```python
from build123d import *

# Parameters (mm, degrees)
SKETCH1_W           = 20
SKETCH1_H           = 15
BOSS_EXTRUDE1_DEPTH = 4.5
SKETCH3_R           = 1.6
CUT_EXTRUDE1_DEPTH  = 20
SKETCH4_W           = 1
SKETCH4_H           = 15
CUT_EXTRUDE2_DEPTH  = 2.5
SKETCH5_W           = 1
SKETCH5_H           = 15
CUT_EXTRUDE3_DEPTH  = 2.5
SKETCH6_W           = 1
SKETCH6_H           = 15
CUT_EXTRUDE5_DEPTH  = 2.5


with BuildPart() as part:
    # Sketch1 → Boss-Extrude1 (new body)
    with BuildSketch(Plane(origin=(0, 0, 0), x_dir=(1, 0, 0), z_dir=(0, 1, 0))):
        Rectangle(SKETCH1_W, SKETCH1_H)
    extrude(amount=BOSS_EXTRUDE1_DEPTH)

    # Sketch3 → Cut-Extrude1 (cut)
    with BuildSketch(Plane(origin=(10, 0, 0), x_dir=(0, 0, -1), z_dir=(1, 0, 0))):
        with Locations((0, 3.72608181)):
            Circle(SKETCH3_R)
    extrude(amount=-CUT_EXTRUDE1_DEPTH, mode=Mode.SUBTRACT)

    # Sketch4 → Cut-Extrude2 (cut)
    with BuildSketch(Plane(origin=(0, 4.5, 0), x_dir=(1, 0, 0), z_dir=(0, 1, 0))):
        with Locations((-7.162357261, 0)):
            Rectangle(SKETCH4_W, SKETCH4_H)
    extrude(amount=-CUT_EXTRUDE2_DEPTH, mode=Mode.SUBTRACT)

    # Sketch5 → Cut-Extrude3 (cut)
    with BuildSketch(Plane(origin=(0, 4.5, 0), x_dir=(1, 0, 0), z_dir=(0, 1, 0))):
        with Locations((-4.526212298, 0)):
            Rectangle(SKETCH5_W, SKETCH5_H)
    extrude(amount=-CUT_EXTRUDE3_DEPTH, mode=Mode.SUBTRACT)

    # Sketch6 → Cut-Extrude5 (cut)
    with BuildSketch(Plane(origin=(0, 4.5, 0), x_dir=(1, 0, 0), z_dir=(0, 1, 0))):
        with Locations((-1.483369352, 0)):
            Rectangle(SKETCH6_W, SKETCH6_H)
    extrude(amount=-CUT_EXTRUDE5_DEPTH, mode=Mode.SUBTRACT)


solid = part.part
```
Here's how the part is built. I have some questions about the finished solid (model axes, mm). A direction names the side the tool comes from. Give positions to 0.01 mm unless a question says otherwise; leave off trailing zeros. Loops run counter-clockwise (first coordinate to the right, second up) from the corner with the lowest first, then second, coordinate; pieces in that order, holes last. Notation, with made-up numbers: M 44,24 L 95,24 A23 ccw 95,34 Z; hole C 66,2 d4. An arc over 180 degrees is marked long. Put each result on its own line as item: value. Start each with the question number.
(1) Will this pin go through, and if not, where does the flat tip stop? pin 1 Ø0.8 at (x, z) = (-1.5, 2) entering from +Y.
(2) I want a section at A-A on z = 5.25. Please give me the cut outline in (x, y), then the cut area to 3 significant figures.
(3) If we mould it in two halves opening along Z, with no side actions, what happens to faces 3 (the flat face through (-7, 2, 0)), 4 (the cylindrical face through (-8.815, 2.127, 0.046))? For each: +Z half, -Z half, draft (parallel to the pull), parting line (faces both ways), or undercut.
(4) I want a section at B-B on y = 4.05. State how many separate pieces and enclosed holes the cut face has, then the cut area to 3 significant figures.
(5) I want a section at C-C on x = 6.25. Please give me the cut outline in (y, z).
(6) I need wall thicknesses on line 1 along X through (y, z) = (3, -5.5); line 2 along Z through (x, y) = (-2.25, 2.95); line 3 along Z through (x, y) = (8, 3.8). Which ranges of each line are inside material? Lowest first, please. Write a range as [from, to].
(7) I want a section at D-D on z = 0. Please give me the cut outline in (x, y).
(8) For faces 1 (the flat face through (-4.5, 2, -0.1)), 2 (the flat face through (10, 1.7, 0.1)), which set-ups out of +Z, -Z, +X, -X, +Y, -Y let a thin tool reach every point of the face, with its end or its side?
Answer block:
1. pin 1: y = 2
2. outline: M -10,0 L 10,0 L 10,4.5 L -0.98,4.5 L -0.98,2 L -1.98,2 L -1.98,4.5 L -4.03,4.5 L -4.03,2 L -5.03,2 L -5.03,4.5 L -6.66,4.5 L -6.66,2 L -7.66,2 L -7.66,4.5 L -10,4.5 Z
2. area: 82.5 mm^2
3. face 3: draft
3. face 4: undercut
4. separate pieces: 8
4. enclosed holes: 0
4. area: 202 mm^2
5. outline: M 0,-7.5 L 4.5,-7.5 L 4.5,-1.4 A1.6 cw long 4.5,1.4 L 4.5,7.5 L 0,7.5 Z
6. line 1: [-10, -7.66], [-6.66, -5.03], [-4.03, -1.98], [-0.98, 10]
6. line 2: [-7.5, -1.4], [1.4, 7.5]
6. line 3: [-7.5, -1.6], [1.6, 7.5]
7. outline: M -10,0 L 10,0 L 10,2.13 L -0.98,2.13 L -0.98,2 L -1.98,2 L -1.98,2.13 L -4.03,2.13 L -4.03,2 L -5.03,2 L -5.03,2.13 L -6.66,2.13 L -6.66,2 L -7.66,2 L -7.66,2.13 L -10,2.13 Z
8. face 1: +Z, -Z, +Y
8. face 2: +Z, -Z, +X, +Y, -Y
